Can you work these out from the model? Positions are in its coordinate system, mm. Face numbers are marked on the shaded views. A direction names the side the tool comes from. Coordinates: 2 decimals unless noted, no trailing zeros. Loops run counter-clockwise (first coordinate to the right, second up) from the corner with the lowest first, then second, coordinate; pieces in that order, holes last. Notation, with made-up numbers: M 15,23 L 47,23 A24 cw 47,53 Z; hole C 27.25,82.5 d4. An arc over 180 degrees is marked long. Return JSON: item names as keys, results as strings. Group by question number.
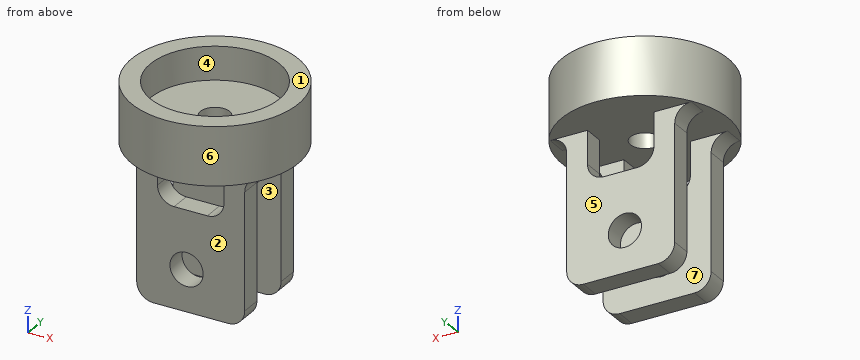
Autodesk Inventor part; units mm, degrees
ref_plane "Work Plane1" through (0, 0, 9.8036) normal (0, 0, 1) x (1, 0, 0)
ref_plane "YZ Plane" through (0, 0, 0) normal (1, 0, 0) x (0, 1, 0)
ref_plane "XZ Plane" through (0, 0, 0) normal (0, 1, 0) x (-1, 0, 0)
sketch "Sketch1" plane through (0, 0, 0) normal (1, 0, 0) x (0, 1, 0)
  line L0 (0, 21.5591) -> (0, -21.8295)
  line L1 (10, 16.8036) -> (0, 16.8036)
  line L2 (0, 16.8036) -> (0, 9.8036)
  line L3 (0, 9.8036) -> (10, 9.8036)
  line L4 (10, 9.8036) -> (10, 16.8036)
  line L5 (5, 9.8036) -> (0, 9.8036)
  line L6 (0, 9.8036) -> (0, -8.1964)
  line L7 (0, -8.1964) -> (5, -8.1964)
  line L8 (5, -8.1964) -> (5, 9.8036)
  line L9 (-5, 9.8036) -> (0, 9.8036)
  line L10 (0, -8.1964) -> (-5, -8.1964)
  line L11 (-5, -8.1964) -> (-5, 9.8036)
  point P0 (0, 0)
  dimension "d0" = 20
  dimension "d1" = 7
  dimension "d5" = 10
  dimension "d7" = 25
revolve "Revolution1" add sketch "Sketch1" angle 360 about axis through (0, 0, 21.5591) along (0, 0, -1) contours L1 L4 L3 L0
extrude "Extrusion1" add sketch "Sketch1" along normal mid plane 13 contours L3 L8 L7 L0 | L0 L10 L11 L9
hole "Hole1" at (0, 0, 16.8036) direction (0, 0, -1) diameter 3.5 end through all counterbore diameter 15.5 counterbore depth 4
ref_plane "Work Plane1" through (0, 0, 9.8036) normal (0, 0, 1) x (1, 0, 0)
sketch "Sketch2" plane through (6.5, 5, -8.1964) normal (0, 0, -1) x (-1, 0, 0)
  circle A0 centre (6.5, -5) radius 1.75
  line L0 (6.5, -5) -> (19.0307, -5)
  line L1 (15.8465, -2.5) -> (-5.7871, -2.5)
  line L2 (-5.7871, -2.5) -> (-5.7871, -7.5)
  line L3 (-5.7871, -7.5) -> (15.8465, -7.5)
  line L4 (15.8465, -7.5) -> (15.8465, -2.5)
  point P0 (6.5, -5)
  dimension "d20" = 5
extrude "Extrusion2" cut sketch "Sketch2" against normal up to surface (18 mm away)
sketch "Sketch3" plane through (0, 0, 9.8036) normal (0, 0, -1) x (-1, 0, 0)
  line L0 (-4, 4) -> (4, 4)
  line L1 (4, 4) -> (4, -4)
  line L2 (4, -4) -> (-4, -4)
  line L3 (-4, -4) -> (-4, 4)
  line L4 (0, 0) -> (0, 10)
  circle A0 centre (0, 0) radius 1.75
  line L5 (0, 0) -> (-11.0224, 0)
  dimension "d33" = 8
extrude "Extrusion3" cut sketch "Sketch3" along normal blind 6 contours L0 L4 A0 L5 L3 | L0 L1 L2 L3 L5 A0 L4
sketch "Sketch4" plane through (-6.5, -5, -8.1964) normal (0, -1, 0) x (1, 0, 0)
  line L0 (0, 18) -> (13, 18)
  line L1 (0, 0) -> (0, 18)
  line L2 (0, 0) -> (13, 0)
  line L3 (13, 18) -> (13, 0)
  circle A0 centre (6, 5) radius 2
  point P0 (6.5, 8.1964)
  dimension "d26" = 5
  dimension "d27" = 4
extrude "Extrusion4" cut sketch "Sketch4" against normal through all contours A0
fillet "Fillet1" radius 2 2 edges at (6.5, -3.75, 9.8036) (6.5, 3.75, 9.8036)
fillet "Fillet1" radius 2 2 edges at (-6.5, -3.75, 9.8036) (-6.5, 3.75, 9.8036)
fillet "Fillet2" radius 2 2 edges at (6.5, 3.75, -8.1964) (-6.5, 3.75, -8.1964)
sketch "Sketch5" plane through (-4, 4, 9.8036) normal (0, -1, 0) x (1, 0, 0)
  line L0 (8, 0) -> (0, 0)
  line L1 (0, 0) -> (0, -6)
  line L2 (0, -6) -> (8, -6)
  line L3 (8, 0) -> (8, -6)
  point P0 (4, -9.8036)
extrude "Extrusion5" cut sketch "Sketch5" along normal through all both and the other way through all
fillet "Fillet3" radius 2 4 edges at (4, -3.75, 3.8036) (4, 3.75, 3.8036) (-4, 3.75, 3.8036) (-4, -3.75, 3.8036)
properties part number "piston"
1) If we mould it in two halves opening along Y, with no side actions, what happens to the marked faces 5, 6 and 7? For each: +Y half, -Y half, draft (parallel to the pull), parting line (faces both ways), or undercut.
2) Suppose I cut it at C-C, the plane z = -0.5. List the corners of the cut face in (x, y) for me, then the cut area to 3 significant figures.
3) Suppose I cut it at A-A, the plane y = 0. List the corners of the cut face in (x, z) for me.
4) If I drill on line 1 (Z direction, x = -0.5, y = 3.15); line 2 (Y direction, x = 3.25, z = 2.5); line 3 (Z direction, x = 5.25, y = 1.5), over which ranges is the centre line in solid material (lowest first)? Write a range as from..to.
5) For the marked faces 1, 2, 3 and 4, which set-ups out of +Z, -Z, +X, -X, +Y, -Y let a thin tool reach every point of the face, with its end or its side?
6) Suppose I cut it at D-D, the plane z = 9.5. List the corners of the cut face in (x, y) for me, then the cut area to 3 significant figures.
7) For pin 1 (0.8 mm diameter, centred on y = 4.5, z = 8.5, fed in from -X); pin 2 (0.8 mm diameter, centred on y = -4, z = 7.5, fed in from -X); pin 3 (5 mm diameter, centred on x = -0.5, z = -3.2, fed in from +Y); pin 4 (3 mm diameter, centred on x = 0, y = 0, fed in from -Z), each with a flat end and sliding along its axis, tell me the tip position at first contact or that it passes through.
8) Suppose I cut it at B-B, the plane x = -0.5. List the corners of the cut face in (y, z) for me.
Returned:
{
 "1": {"face 5": "+Y half", "face 6": "parting line", "face 7": "undercut"},
 "2": {"outline": "M -6.5,-5 L 6.5,-5 L 6.5,-2.5 L -6.5,-2.5 Z; M -6.5,2.5 L 6.5,2.5 L 6.5,5 L -6.5,5 Z", "area": "65.0 mm²"},
 "3": {"outline": "M -10,9.8 L -1.75,9.8 L -1.75,12.8 L -7.75,12.8 L -7.75,16.8 L -10,16.8 Z; M 1.75,9.8 L 10,9.8 L 10,16.8 L 7.75,16.8 L 7.75,12.8 L 1.75,12.8 Z"},
 "4": {"line 1": "z = -8.2..-5.2, -1.2..3.8, 9.8..12.8", "line 2": "y = -5..-2.5, 2.5..5", "line 3": "z = 9.8..12.8"},
 "5": {"face 1": "+Z, +X, -X, +Y, -Y", "face 2": "-Z, +X, -X, -Y", "face 3": "-Z, +X, -X", "face 4": "+Z"},
 "6": {"outline": "M -7.44,-5 L -4,-5 L -4,-2.5 L -7.44,-2.5 Z; M -7.44,2.5 L -4,2.5 L -4,5 L -7.44,5 Z; M 4,-5 L 7.44,-5 L 7.44,-2.5 L 4,-2.5 Z; M 4,2.5 L 7.44,2.5 L 7.44,5 L 4,5 Z", "area": "34.4 mm²"},
 "7": {"pin 1": "stops at x = -6.83", "pin 2": "stops at x = -6.5", "pin 3": "stops at y = 5", "pin 4": "passes through"},
 "8": {"outline": "M -9.99,9.8 L -1.68,9.8 L -1.68,12.8 L -7.73,12.8 L -7.73,16.8 L -9.99,16.8 Z; M -5,-8.2 L -2.5,-8.2 L -2.5,-5.2 L -5,-5.2 Z; M -5,-1.2 L -2.5,-1.2 L -2.5,3.8 L -5,3.8 Z; M 1.68,9.8 L 9.99,9.8 L 9.99,16.8 L 7.73,16.8 L 7.73,12.8 L 1.68,12.8 Z; M 2.5,-8.2 L 5,-8.2 L 5,-5.2 L 2.5,-5.2 Z; M 2.5,-1.2 L 5,-1.2 L 5,3.8 L 2.5,3.8 Z"}
}
